Geometry check sheet. Reference: drawing and pictorial views, mm from the part's lowest x, y, z. A direction names the side the tool comes from. Give positions to 0.01 mm unless a question says otherwise; leave off trailing zeros. Order: outer loops, then holes, each group sorted by start corner. A loop starts at its lowest first (then second) coordinate and runs counter-clockwise, first axis right, second up.
Item 1: Access from +Z, -Z, +X, -X, +Y, -Y to the whole of each face (thin tool, end or side, straight path). Record for the marked faces 1 and 2.
Item 2: Material ranges on line 1 along Y through (x, z) = (7, 7); line 2 along Y through (x, z) = (11.25, 10.25); line 3 along X through (y, z) = (46, 7), recorded low to high.
Item 3: Sectioned sample at C-C on y = 46. Record the boundary of the cut face in (x, z).
Item 4: Sectioned sample at A-A on x = 7. Record the boundary of the cut face in (y, z).
Item 5: Sectioned sample at D-D on y = 9. Record the boundary of the cut face in (x, z).
Item 6: Gauge pin test, flat end, axial feed: P1, Ø1.5, axis at x = 10.5, y = 8.5, coming from the -Z side. Record the tip position at first contact, or that the pin passes through.
Item 7: Sectioned sample at B-B on z = 7. Record the boundary of the cut face in (x, y).
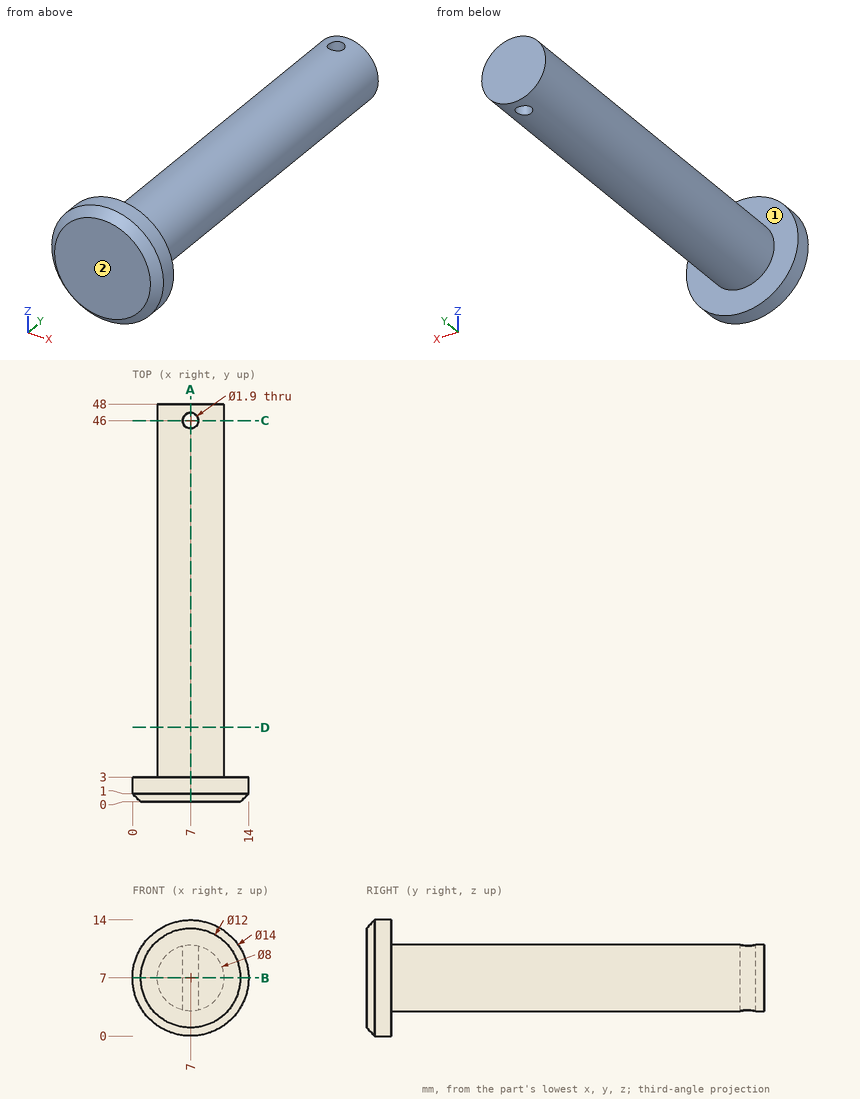
Report:
1. face 1: +Y
1. face 2: +Z, -Z, +X, -X, -Y
2. line 1: y = 0 to 45.05, 46.95 to 48
2. line 2: y = 0 to 3
2. line 3: x = 3 to 6.05, 7.95 to 11
3. outline: (6.05, 3.11) - (6.05, 10.89) arc R4 ccw to start; (7.95, 3.11) arc R4 ccw to (7.95, 10.89) - close
4. outline: (0, 1) - (1, 0) - (3, 0) - (3, 3) - (45.05, 3) - (45.05, 11) - (3, 11) - (3, 14) - (1, 14) - (0, 13) - close; (46.95, 3) - (48, 3) - (48, 11) - (46.95, 11) - close
5. outline: circle Ø8 at (7, 7)
6. P1: stops at z = 4.1
7. outline: (0, 1) - (1, 0) - (13, 0) - (14, 1) - (14, 3) - (11, 3) - (11, 48) - (3, 48) - (3, 3) - (0, 3) - close; hole circle Ø1.9 at (7, 46)
